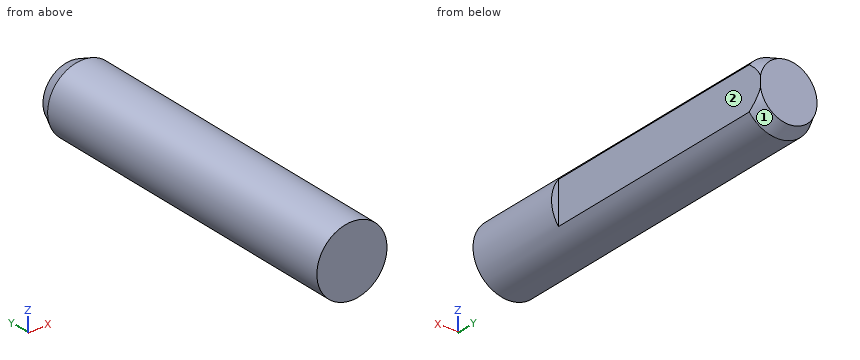
```python
from build123d import *

# Parameters (mm, degrees)
SKETCH_1_R          = 2.5
EXTRUDE_1_DEPTH     = 25
CUT_EXTRUDE_1_DEPTH = 18
CHAMFER_1_SIZE      = 1
CHAMFER_1_SIZE2     = 0.466307658


with BuildPart() as part:
    # 草图1 → 凸台-拉伸1 (new body)
    with BuildSketch(Plane(origin=(0, 0, 0), x_dir=(1, 0, 0), z_dir=(0, 1, 0))):
        Circle(SKETCH_1_R)
    extrude(amount=EXTRUDE_1_DEPTH)

    # 草图2 → 切除-拉伸1 (cut)
    with BuildSketch(Plane(origin=(0, 25, 0), x_dir=(1, 0, 0), z_dir=(0, 1, 0))):
        Polygon((2, 2.598987806), (2, -2.361624848), (2.93708026, -2.012796341), (3.777563327, -1.758131015), (3.87416052, -0.748251275), align=None)
    extrude(amount=-CUT_EXTRUDE_1_DEPTH, mode=Mode.SUBTRACT)

    # 倒角1
    chamfer_1_edges = [part.edges().sort_by_distance(p)[0] for p in [
        (-2.5, 25, 0),
    ]]
    chamfer_1_side = [part.faces().sort_by_distance(p)[0] for p in [
        (-2.5, 12.5, 0),
    ]]
    chamfer(chamfer_1_edges, length=CHAMFER_1_SIZE, length2=CHAMFER_1_SIZE2, reference=chamfer_1_side[0])


solid = part.part
```
Design review of the part built by this model. Coordinates are the model's own, in mm. Face numbers are marked on the shaded views. A direction names the side the tool comes from. Give positions to 0.01 mm unless a question says otherwise; leave off trailing zeros. Loops run counter-clockwise (first coordinate to the right, second up) from the corner with the lowest first, then second, coordinate; pieces in that order, holes last. Notation, with made-up numbers: (52, 47) -> (98, 47) arc R13 cw to (98, 58) -> close; hole circle Ø2 at (68, 21). An arc over 180 degrees is marked (long way). One line per item, written item: value.
Q1. We need section A-A on z = 0. Give the boundary of the cut face in (x, y), and give its area (3 significant figures).
Numbers:
outline: (-2.5, 0) -> (2.5, 0) -> (2.5, 7) -> (2, 7) -> (2, 25) -> (-2.03, 25) -> (-2.5, 24) -> close
area: 116 mm^2
Q2. For L1, parallel to X at y = 2.5, z = 2; L2, parallel to X at y = 14.75, z = -0.15; L3, parallel to Y at x = -1.15, z = 2, list the stretches that pass through material, from the lowest coordinate up.
Numbers:
L1: x = -1.5 to 1.5
L2: x = -2.5 to 2
L3: y = 0 to 24.41
Q3. We need section C-C on y = 4.75. Give the boundary of the cut face in (x, z).
Numbers:
outline: circle Ø5 at (0, 0)
Q4. We need section B-B on y = 10.5. Give the boundary of the cut face in (x, z).
Numbers:
outline: (2, -1.5) -> (2, 1.5) arc R2.5 ccw (long way) to start
Q5. For pin 1 Ø2 at (y, z) = (9, -1) entering from +X; pin 2 Ø1.5 at (x, y) = (-1, 18.5) entering from +Z, all flat-tipped, find the tip position at first contact; note any pin that passes through.
Numbers:
pin 1: stops at x = 2
pin 2: stops at z = 2.49
Q6. Machinability: for the marked faces 1 and 2, which of the approach directions +Z, -Z, +X, -X, +Y, -Y give a long, thin tool a straight path to every point of the face, cutting with its end or side? Answer none if there is none.
Numbers:
face 1: +Y
face 2: +Z, -Z, +X, +Y
